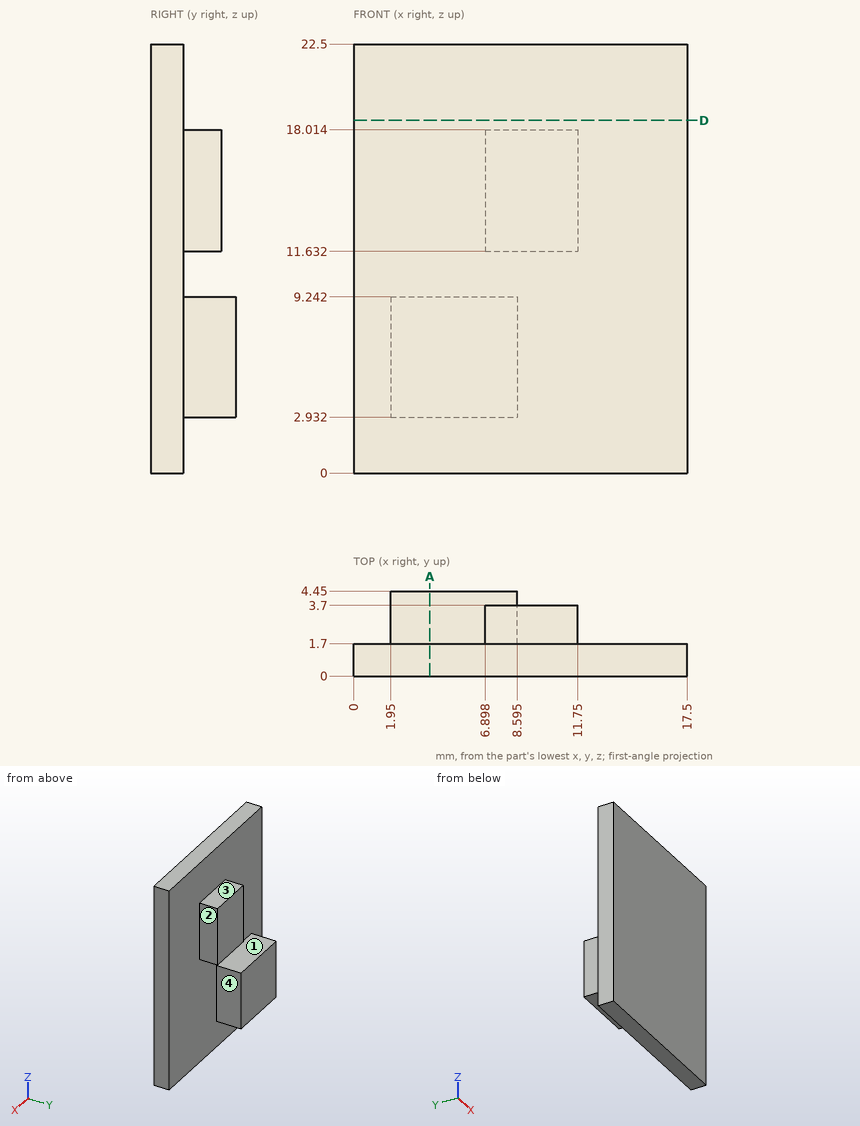
Check sheet for the drawn part. Datum: minimum x, y, z corner. Units: mm. A direction names the side the tool comes from. Give positions to 0.01 mm unless a question says otherwise; leave off trailing zeros. Write each loop counter-clockwise with the first axis right and the second up, starting at its lowest first coordinate (ties: lowest second). Pieces come first, ordered by that corner, then holes. Notation, with made-up numbers: (-0.5, -23) - (54.5, -23) arc R22 cw to (54.5, -9) - close; hole circle Ø9 at (-26, 27.25). An arc over 180 degrees is marked (long way). Put each result on its own line as item: value.
1. Sectioned sample at D-D, the plane z = 18.5. Enter the section's corners in (x, y).
Ans:
outline: (0, 0) - (17.5, 0) - (17.5, 1.7) - (0, 1.7) - close
2. Set-up check for the marked faces 1, 2, 3 and 4: record each of +Z, -Z, +X, -X, +Y, -Y from which the full face is reachable in a straight line by a thin tool's end or side.
Ans:
face 1: +X, -X, +Y
face 2: +Z, -Z, +X, +Y
face 3: +Z, +X, -X, +Y
face 4: -Z, +X, +Y
3. Thickness scan on line 1 (Y direction, x = 8, z = 10.75); line 2 (Z direction, x = 6.5, y = 3.2); line 3 (Z direction, x = 11.5, y = 2.8) (1 decimal). Record the ranges inside material, lowest first.
Ans:
line 1: y = 0 to 1.7
line 2: z = 2.93 to 9.24
line 3: z = 11.6 to 18
4. Sectioned sample at A-A, the plane x = 4. Enter the section's corners in (y, z).
Ans:
outline: (0, 0) - (1.7, 0) - (1.7, 2.93) - (4.45, 2.93) - (4.45, 9.24) - (1.7, 9.24) - (1.7, 22.5) - (0, 22.5) - close
5. Go/stop test with flat-tipped pins: pin 1 (1.5 mm diameter, centred on x = 10, z = 14.5, fed in from +Y); pin 2 (2 mm diameter, centred on x = 10, y = 3, fed in from -Z); pin 3 (1.6 mm diameter, centred on x = 10, y = 3, fed in from +Z) (1 decimal). Record where each tip stops, or that it passes through.
Ans:
pin 1: stops at y = 3.7
pin 2: stops at z = 11.63
pin 3: stops at z = 18
